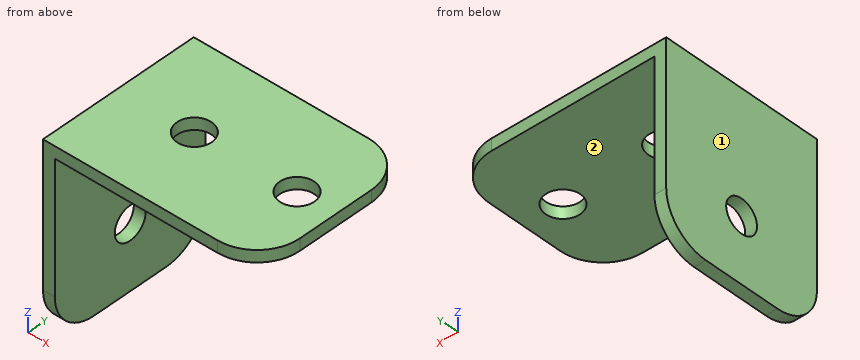
from build123d import *

# Parameters (mm, degrees)
BOSS_EXTRUDE1_DEPTH = 38.1
FILLET1_R           = 10
SKETCH2_R           = 4.05
CUT_EXTRUDE1_DEPTH  = 3.75336
SKETCH3_R           = 3.893907584
CUT_EXTRUDE2_DEPTH  = 3.75336


with BuildPart() as part:
    # Sketch1 → Boss-Extrude1 (new body)
    with BuildSketch(Plane(origin=(0, 0, 0), x_dir=(1, 0, 0), z_dir=(0, 1, 0))):
        Polygon((-25.4, -21.59), (25.4, -21.59), (25.4, -18.83664), (-22.64664, -18.83664), (-22.64664, 21.59), (-25.4, 21.59), align=None)
    extrude(amount=BOSS_EXTRUDE1_DEPTH)

    # Fillet1
    fillet1_edges = [part.edges().sort_by_distance(p)[0] for p in [
        (25.4, 38.1, 20.21332),
        (-24.02332, 38.1, -21.59),
        (-24.02332, 0, -21.59),
        (25.4, 0, 20.21332),
    ]]
    fillet(fillet1_edges, radius=FILLET1_R)

    # Sketch2 → Cut-Extrude1 (cut, through all)
    with BuildSketch(Plane(origin=(0, 0, 18.83664), x_dir=(-1, 0, 0), z_dir=(0, 0, -1))):
        with Locations((-16.35336, 19.05)):
            Circle(SKETCH2_R)
        with Locations((7.64664, 19.05)):
            Circle(SKETCH2_R)
    extrude(amount=-CUT_EXTRUDE1_DEPTH, mode=Mode.SUBTRACT)

    # Sketch3 → Cut-Extrude2 (cut, through all)
    with BuildSketch(Plane(origin=(-22.64664, 0, 0), x_dir=(0, 0, -1), z_dir=(1, 0, 0))):
        with Locations((6.56336, 19.05)):
            Circle(SKETCH3_R)
    extrude(amount=-CUT_EXTRUDE2_DEPTH, mode=Mode.SUBTRACT)


solid = part.part
Work out the finished part from the listing and answer in its coordinate system (mm). Face numbers are marked on the shaded views. A direction names the side the tool comes from. Give positions to 0.01 mm unless a question says otherwise; leave off trailing zeros. Order: outer loops, then holes, each group sorted by start corner. A loop starts at its lowest first (then second) coordinate and runs counter-clockwise, first axis right, second up. Notation, with made-up numbers: (23, 84) -> (40, 84) arc R23 ccw to (40, 121) -> close; hole circle Ø10 at (-1.5, -30.75). An arc over 180 degrees is marked (long way). Answer as a JSON object with one key per item and string values. Group by question number.
1. Section B-B on z = -7 is taken. Determine the outline of the cut face in (x, y), plus the area to 3 significant figures.
2. Flat-ended cylindrical pins translate along their axes: pin 1 Ø10 at (y, z) = (19.05, -6.56) entering from +X; pin 2 Ø3 at (x, y) = (4, 32) entering from -Z. Find the tip coordinate at first contact, or state that the pin passes through.
3. Consider line 1 along X through (y, z) = (27.5, -18.5); line 2 along Z through (x, y) = (21.5, 22.5). Determine where each line is inside the solid, lowest interval first. Write a range as [from, to].
4. Section A-A on y = 19.05 is taken. Determine the outline of the cut face in (x, z).
5. Section D-D on z = 6 is taken. Determine the outline of the cut face in (x, y).
6. Section C-C on x = 2.5 is taken. Determine the outline of the cut face in (y, z), plus the area to 3 significant figures.
7. A tool of negligible diameter and unlimited length cuts with its end or side. For the marked faces 1 and 2, from which of +Z, -Z, +X, -X, +Y, -Y can it reach the whole face along a straight path? Write none if from no direction.
Result sheet:
{
 "1": {"outline": "(-25.4, 0) -> (-22.65, 0) -> (-22.65, 15.18) -> (-25.4, 15.18) -> close; (-25.4, 22.92) -> (-22.65, 22.92) -> (-22.65, 38.1) -> (-25.4, 38.1) -> close", "area": "83.6 mm^2"},
 "2": {"pin 1": "stops at x = -22.65", "pin 2": "stops at z = 18.84"},
 "3": {"line 1": "x = [-25.4, -22.65]", "line 2": "z = [18.84, 21.59]"},
 "4": {"outline": "(-25.4, -21.59) -> (-22.65, -21.59) -> (-22.65, -10.46) -> (-25.4, -10.46) -> close; (-25.4, -2.67) -> (-22.65, -2.67) -> (-22.65, 18.84) -> (-11.7, 18.84) -> (-11.7, 21.59) -> (-25.4, 21.59) -> close; (-3.6, 18.84) -> (12.3, 18.84) -> (12.3, 21.59) -> (-3.6, 21.59) -> close; (20.4, 18.84) -> (25.4, 18.84) -> (25.4, 21.59) -> (20.4, 21.59) -> close"},
 "5": {"outline": "(-25.4, 0) -> (-22.65, 0) -> (-22.65, 38.1) -> (-25.4, 38.1) -> close"},
 "6": {"outline": "(0, 18.84) -> (38.1, 18.84) -> (38.1, 21.59) -> (0, 21.59) -> close", "area": "105 mm^2"},
 "7": {"face 1": "+Z, -Z, -X, +Y, -Y", "face 2": "-Z, +X, +Y, -Y"}
}
